from build123d import *

# Parameters (mm, degrees)
F0_W      = 20
F0_H      = 20
F1_DEPTH  = 10
F5_R      = 0.748055
F6_DEPTH  = 2
F7_R      = 0.641611
F8_DEPTH  = 2
F9_R      = 0.67615
F10_DEPTH = 2


with BuildPart() as f1:
    # F0 (on Front) → F1 (new body, symmetric)
    with BuildSketch(Plane.XZ):
        Rectangle(F0_W, F0_H)
    extrude(amount=F1_DEPTH, both=True)

    # F2 (on Front) → F3 (revolve, intersect)
    with BuildSketch(Plane.XZ):
        with BuildLine():
            Line((0, -13.830679), (0, 13.830679))
            ThreePointArc((0, 13.830679), (-13.830679, 0), (0, -13.830679))
        make_face()
    revolve(axis=Axis((0, 0, 1.024824), (0, 0, 1)), mode=Mode.INTERSECT)

    # F5 (on face) → F6 (cut)
    with BuildSketch(Plane.YZ.offset(10)):
        with Locations((0, -5.701799)):
            Circle(F5_R)
        with Locations((-5.701799, -5.701799)):
            Circle(F5_R)
        with Locations((-5.701799, 0)):
            Circle(F5_R)
        with Locations((-5.701799, 5.701799)):
            Circle(F5_R)
        with Locations((0, 5.701799)):
            Circle(F5_R)
        with Locations((5.701799, 5.701799)):
            Circle(F5_R)
        with Locations((5.701799, 0)):
            Circle(F5_R)
    extrude(amount=-F6_DEPTH, mode=Mode.SUBTRACT)

    # F7 (on face) → F8 (cut)
    with BuildSketch(Plane.XZ.offset(10)):
        with Locations((-5.701799, 5.701799)):
            Circle(F7_R)
        with Locations((-5.701799, 0.41338)):
            Circle(F7_R)
        with Locations((-5.701799, -5.701799)):
            Circle(F7_R)
        with Locations((0, -5.701799)):
            Circle(F7_R)
        with Locations((5.701799, -5.701799)):
            Circle(F7_R)
        with Locations((5.701799, 0)):
            Circle(F7_R)
        with Locations((5.701799, 5.701799)):
            Circle(F7_R)
        with Locations((0, 5.701799)):
            Circle(F7_R)
    extrude(amount=-F8_DEPTH, mode=Mode.SUBTRACT)

    # F9 (on face) → F10 (cut)
    with BuildSketch(Plane(origin=(-10, 0, 0), x_dir=(0, -1, 0), z_dir=(-1, 0, 0))):
        with Locations((-0.299345, 5.701799)):
            Circle(F9_R)
        with Locations((-5.701799, 5.701799)):
            Circle(F9_R)
        with Locations((-5.701799, 0)):
            Circle(F9_R)
        with Locations((-5.701799, -5.701799)):
            Circle(F9_R)
        with Locations((0, -5.701799)):
            Circle(F9_R)
        with Locations((5.701799, -5.701799)):
            Circle(F9_R)
        with Locations((5.701799, 0)):
            Circle(F9_R)
        with Locations((5.701799, 5.701799)):
            Circle(F9_R)
    extrude(amount=-F10_DEPTH, mode=Mode.SUBTRACT)


solid = f1.part
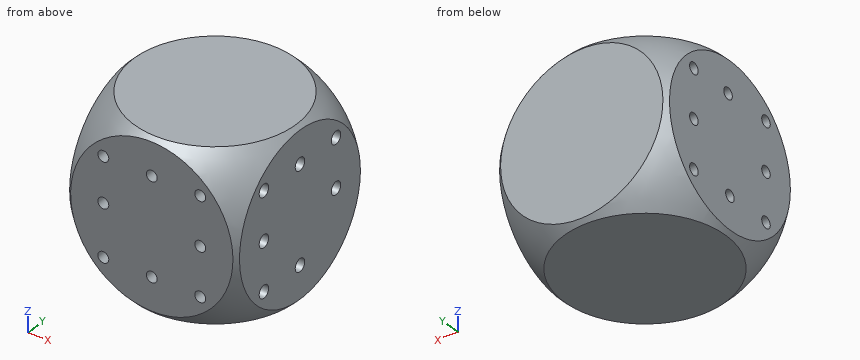
Design review of the part built by this model. Coordinates are the model's own, in mm. Give positions to 0.01 mm unless a question says otherwise; leave off trailing zeros. Order: outer loops, then holes, each group sorted by start corner. A loop starts at its lowest first (then second) coordinate and runs counter-clockwise, first axis right, second up. Notation, with made-up numbers: (63.5, 88) - (85.5, 88) arc R5 ccw to (85.5, 95) - close; hole circle Ø6 at (82.25, -8.5). An arc over 180 degrees is marked (long way). Write item = value, one per line. Start each with the question number.
Q1. To check wall thickness, follow L1, parallel to Z at x = 9.3, y = 0; L2, parallel to Y at x = -8.5, z = -0.25; L3, parallel to Y at x = -4.5, z = 9.25. State the ranges of each line that lie inside material, in increasing order. Write a range as from..to.
Q2. We need section C-C on y = 0. State the section outline as (x, z) points, plus the area to 3 significant figures.
Q3. We need section B-B on y = 7.5. State the section outline as (x, z) points.
Q4. We need section A-A on z = 7. State the section outline as (x, y) points.
Q5. Clearance check with a flat-ended pin moving along its axis: pin 1 Ø0.7 at (y, z) = (-5.5, 6) entering from +X. State where the tip first meets the part, or that it passes through.
Working result:
q1.L1 = -10..-6.45, -4.95..4.95, 6.45..10
q1.L2 = -10..-6.33, -5.07..5.07, 6.33..10
q1.L3 = -9.25..9.25
q2.outline = (-10, -9.55) arc R13.83 ccw to (-9.55, -10) - (9.55, -10) arc R13.83 ccw to (10, -9.55) - (10, -6.45) - (8, -6.45) - (8, -4.95) - (10, -4.95) - (10, 4.95) - (8, 4.95) - (8, 6.45) - (10, 6.45) - (10, 9.55) arc R13.83 ccw to (9.55, 10) - (-9.55, 10) arc R13.83 ccw to (-10, 9.55) - (-10, 6.31) - (-8, 6.31) - (-8, 5.1) - (-10, 5.1) - (-10, -5.03) - (-8, -5.03) - (-8, -6.38) - (-10, -6.38) - close
q2.area = 388 mm²
q3.outline = (-10, -5.92) arc R11.62 ccw to (-5.92, -10) - (5.92, -10) arc R11.62 ccw to (10, -5.92) - (10, 5.92) arc R11.62 ccw to (5.92, 10) - (-5.92, 10) arc R11.62 ccw to (-10, 5.92) - close
q4.outline = (-10, -6.5) arc R11.93 ccw to (-6.5, -10) - (6.5, -10) arc R11.93 ccw to (10, -6.5) - (10, 6.5) arc R11.93 ccw to (6.5, 10) - (-6.5, 10) arc R11.93 ccw to (-10, 6.5) - close
q5.pin_1 = 8
